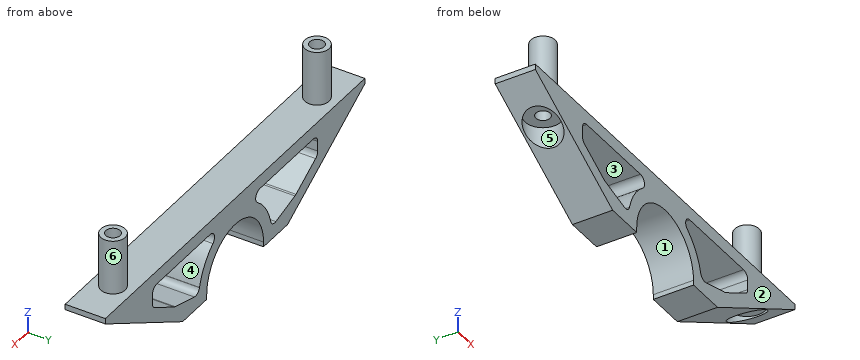
from build123d import *

# Parameters (mm, degrees)
F1_DEPTH = 9.525
F3_R     = 8.4582
F4_DEPTH = 27.45994
F6_R     = 5.7785
F7_DEPTH = 25.908
F8_R     = 3.4036
F9_DEPTH = 76.2


with BuildPart() as f1:
    # F0 (on Front) → F1 (new body, symmetric)
    with BuildSketch(Plane.XZ):
        with BuildLine():
            Line((21.6535, 0), (40.005, 0))
            Line((40.005, 0), (98.9457, 34.0294290112))
            Line((98.9457, 34.0294290112), (98.9457, 36.68776))
            Line((98.9457, 36.68776), (-98.9457, 36.68776))
            Line((-98.9457, 36.68776), (-98.9457, 34.0294290112))
            Line((-98.9457, 34.0294290112), (-40.005, 0))
            Line((-40.005, 0), (-21.6535, 0))
            Line((-21.6535, 0), (-21.6535, 2.33426))
            ThreePointArc((-21.6535, 2.33426), (0, 23.98776), (21.6535, 2.33426))
            Line((21.6535, 2.33426), (21.6535, 0))
        make_face()
        with BuildLine():
            Line((-59.8033378542, 30.33776), (-18.8585378542, 30.33776))
            ThreePointArc((-18.8585378542, 30.33776), (-15.8495372268, 28.1759432135), (-16.9381164842, 24.6343995112))
            ThreePointArc((-16.9381164842, 24.6343995112), (-23.3636326477, 17.7724166824), (-27.1562111419, 9.170648569))
            ThreePointArc((-27.1562111419, 9.170648569), (-27.1707416417, 9.1098353716), (-27.1864668557, 9.0493201004))
            ThreePointArc((-27.1864668557, 9.0493201004), (-28.6668651927, 7.1267195186), (-31.072771318, 6.8111439337))
            Line((-31.072771318, 6.8111439337), (-45.649831318, 10.7151239337))
            ThreePointArc((-45.649831318, 10.7151239337), (-46.0432879059, 10.848642966), (-46.4159399977, 11.0323977948))
            Line((-46.4159399977, 11.0323977948), (-61.3917799977, 19.6785577948))
            ThreePointArc((-61.3917799977, 19.6785577948), (-62.5539248829, 20.8406899989), (-62.9793, 22.4282))
            Line((-62.9793, 22.4282), (-62.9793, 27.16276))
            ThreePointArc((-62.9793, 27.16276), (-62.0490238861, 29.4081642686), (-59.8033378542, 30.33776))
        make_face(mode=Mode.SUBTRACT)
        with BuildLine():
            ThreePointArc((31.072771318, 6.8111439337), (28.6668651927, 7.1267195186), (27.1864668557, 9.0493201004))
            ThreePointArc((27.1864668557, 9.0493201004), (27.1707416417, 9.1098353716), (27.1562111419, 9.170648569))
            ThreePointArc((27.1562111419, 9.170648569), (23.3636326477, 17.7724166824), (16.9381164842, 24.6343995112))
            ThreePointArc((16.9381164842, 24.6343995112), (15.8495372268, 28.1759432135), (18.8585378542, 30.33776))
            Line((18.8585378542, 30.33776), (59.8033378542, 30.33776))
            ThreePointArc((59.8033378542, 30.33776), (62.0490238861, 29.4081642686), (62.9793, 27.16276))
            Line((62.9793, 27.16276), (62.9793, 22.4282))
            ThreePointArc((62.9793, 22.4282), (62.5539248829, 20.8406899989), (61.3917799977, 19.6785577948))
            Line((61.3917799977, 19.6785577948), (46.4159399977, 11.0323977948))
            ThreePointArc((46.4159399977, 11.0323977948), (46.0432879059, 10.848642966), (45.649831318, 10.7151239337))
            Line((45.649831318, 10.7151239337), (31.072771318, 6.8111439337))
        make_face(mode=Mode.SUBTRACT)
    extrude(amount=F1_DEPTH, both=True)

    # F3 (on offset) → F4 (cut)
    with BuildSketch(Plane(origin=(0, 0, 0), x_dir=(1, 0, 0), z_dir=(0, 0, -1))):
        with Locations((-77.7875, 0)):
            Circle(F3_R)
        with Locations((77.7875, 0)):
            Circle(F3_R)
    extrude(amount=-F4_DEPTH, mode=Mode.SUBTRACT)

    # F6 (on offset) → F7 (join)
    with BuildSketch(Plane.XY.offset(36.68776)):
        with Locations((-77.7875, 0)):
            Circle(F6_R)
        with Locations((77.7875, 0)):
            Circle(F6_R)
    extrude(amount=F7_DEPTH)

    # F8 (on offset) → F9 (cut)
    with BuildSketch(Plane(origin=(0, 0, 0), x_dir=(1, 0, 0), z_dir=(0, 0, -1))):
        with Locations((-77.7875, 0)):
            Circle(F8_R)
        with Locations((77.7875, 0)):
            Circle(F8_R)
    extrude(amount=-F9_DEPTH, mode=Mode.SUBTRACT)


solid = f1.part
Could you check a few things on this model? Use its own coordinates, in mm. Face numbers are marked on the shaded views. A direction names the side the tool comes from. Give positions to 0.01 mm unless a question says otherwise; leave off trailing zeros. Write each loop counter-clockwise with the first axis right and the second up, starting at its lowest first coordinate (ties: lowest second). Pieces come first, ordered by that corner, then holes. Notation, with made-up numbers: (-10, 87.5) -> (13, 87.5) arc R17 ccw to (13, 93.5) -> close; hole circle Ø9 at (-23, -32). An arc over 180 degrees is marked (long way). Answer as a JSON object with one key per item and string values.
Q1. We'd pull the mould along Z, two halves only. Please class the marked faces 1, 2 and 3: released by +Z, released by -Z, zero draft, split by the parting line, or undercut.
Taken from the geometry:
{"face 1": "released by -Z", "face 2": "zero draft", "face 3": "undercut"}
Q2. Will these pins go through, and if not, where does the flat tip stop? pin 1 Ø8 at (x, z) = (51, 28) entering from +Y (3 decimals); pin 2 Ø5 at (y, z) = (-3.5, 25.5) entering from +X; pin 3 Ø2.5 at (y, z) = (3, 1) entering from -X; pin 4 Ø1.2 at (y, z) = (2.5, 1.5) entering from +X.
Taken from the geometry:
{"pin 1": "stops at y = 9.525", "pin 2": "stops at x = 88.5", "pin 3": "stops at x = -43.9", "pin 4": "stops at x = 43.64"}
Q3. Suppose I cut it at D-D on y = 0. Count the separate pieces of the cut face and the enclosed holes in it, then the cut area to 3 significant figures.
Taken from the geometry:
{"separate pieces": "3", "enclosed holes": "2", "area": "2,790 mm²"}
Q4. Suppose I cut it at C-C on z = 14. Write out the boundary of the cut face in (x, y) (3 decimals), then the cut area to 3 significant figures.
Taken from the geometry:
{"outline": "(-64.254, -9.525) -> (-51.556, -9.525) -> (-51.556, 9.525) -> (-64.254, 9.525) -> close; (-25.458, -9.525) -> (-18.242, -9.525) -> (-18.242, 9.525) -> (-25.458, 9.525) -> close; (18.242, -9.525) -> (25.458, -9.525) -> (25.458, 9.525) -> (18.242, 9.525) -> close; (51.556, -9.525) -> (64.254, -9.525) -> (64.254, 9.525) -> (51.556, 9.525) -> close", "area": "759 mm²"}
Q5. Which directions (+Z, -Z, +X, -X, +Y, -Y) give clear straight access to the entire face, cutting with the end or side of a thin tool? Please do the marked faces 4, 5 and 6.
Taken from the geometry:
{"face 4": "+Y, -Y", "face 5": "-Z", "face 6": "+Z"}
Q6. Please list where these lines run through material, in increasing order: L1, parallel to X at y = 0, z = 25; L2, parallel to X at y = 0, z = 22.25; L3, parallel to X at y = -4.75, z = 18.
Taken from the geometry:
{"L1": "x = -69.33 to -62.98, -16.53 to 16.53, 62.98 to 69.33", "L2": "x = -69.33 to -62.97, -19.69 to -8.5, 8.5 to 19.69, 62.97 to 69.33", "L3": "x = -70.79 to -58.48, -23.21 to -14.95, 14.95 to 23.21, 58.48 to 70.79"}
Q7. Suppose I cut it at A-A on z = 56. Write out the boundary of the cut face in (x, y).
Taken from the geometry:
{"outline": "circle Ø11.56 at (-77.79, 0); circle Ø11.56 at (77.79, 0); hole circle Ø6.81 at (-77.79, 0); hole circle Ø6.81 at (77.79, 0)"}
Q8. Suppose I cut it at B-B on x = 79.5. Write out the boundary of the cut face in (y, z) (3 decimals).
Taken from the geometry:
{"outline": "(-9.525, 22.802) -> (-8.283, 22.802) -> (-8.283, 27.46) -> (-2.941, 27.46) -> (-2.941, 62.596) -> (-5.519, 62.596) -> (-5.519, 36.688) -> (-9.525, 36.688) -> close; (2.941, 27.46) -> (8.283, 27.46) -> (8.283, 22.802) -> (9.525, 22.802) -> (9.525, 36.688) -> (5.519, 36.688) -> (5.519, 62.596) -> (2.941, 62.596) -> close"}
